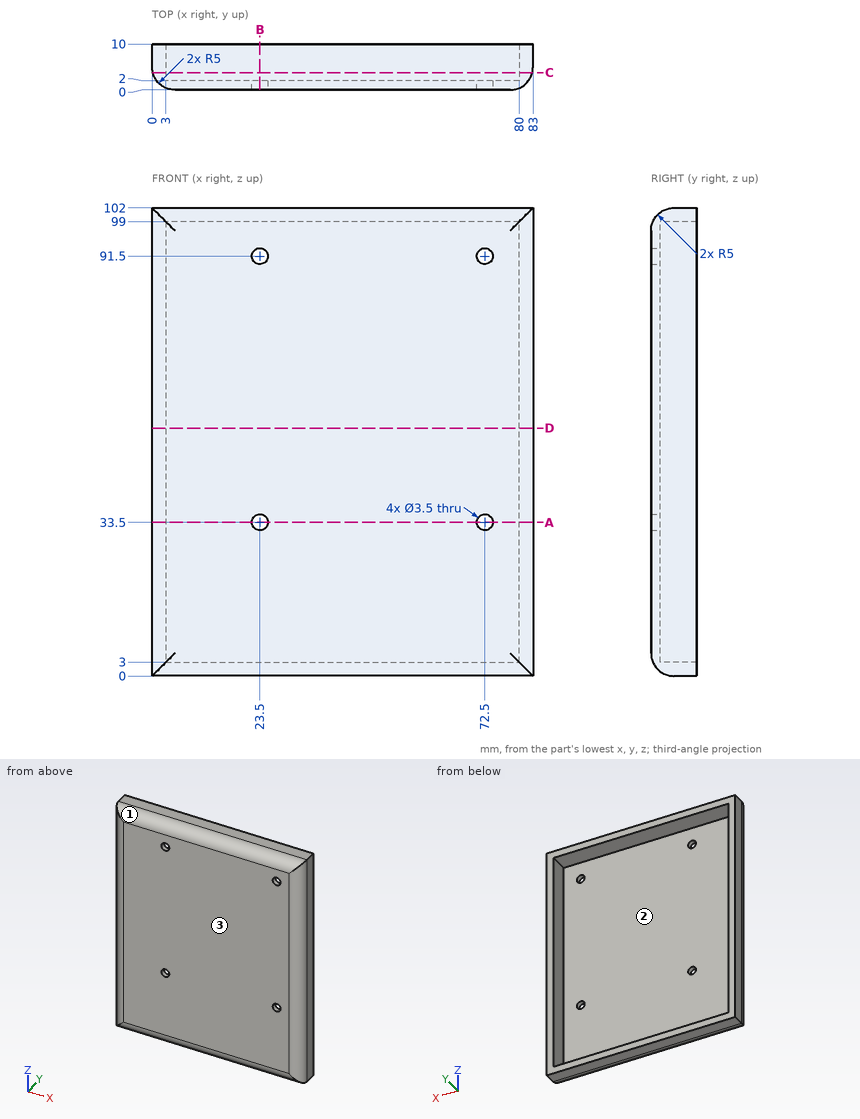
Check sheet for the drawn part. Datum: minimum x, y, z corner. Units: mm. Round coordinates to 2 decimals unless told otherwise and drop trailing zeros. Loops run counter-clockwise (first coordinate to the right, second up) from the corner with the lowest first, then second, coordinate; pieces in that order, holes last. Notation, with made-up numbers: (-2.75, 23) -> (53.25, 23) arc R36 ccw to (53.25, 62) -> close; hole circle Ø4 at (20.25, 1). An arc over 180 degrees is marked (long way). Put each result on its own line as item: value. Start each with the question number.
1. Section check B-B (x = 23.5). Enter the section's corners in (y, z), plus the area to 3 significant figures.
2. Gauge pin test, flat ends, axial feed: pin 1 (3 mm diameter, centred on x = 72.5, z = 91.5, fed in from -Y); pin 2 (5.5 mm diameter, centred on x = 23.5, z = 33.5, fed in from +Y); pin 3 (2 mm diameter, centred on y = 1, z = 86, fed in from +X); pin 4 (3 mm diameter, centred on x = 22.5, y = 3, fed in from -Z). Record the tip position at first contact, or that the pin passes through.
3. Section check D-D (z = 54). Enter the section's corners in (x, y), plus the area to 3 significant figures.
4. Section check C-C (y = 3.75). Enter the section's corners in (x, z), plus the area to 3 significant figures.
5. Draft check along Z on the marked faces 1, 2 and 3. Enter one of: +Z half, -Z half, draft (parallel to the pull), parting line (faces both ways), or undercut.
6. Scan lines: probe 1 along X at (y, z) = (7.75, 7); probe 2 along Z at (x, y) = (64, 8.75); probe 3 along Z at (x, y) = (72.5, 1.65). Record each from-to range of solid material in increasing order.
7. Section check A-A (z = 33.5). Enter the section's corners in (x, y), plus the area to 3 significant figures.
Findings:
1. outline: (0, 5) arc R5 ccw to (5, 0) -> (10, 0) -> (10, 3) -> (2, 3) -> (2, 31.75) -> (0, 31.75) -> close; (0, 35.25) -> (2, 35.25) -> (2, 89.75) -> (0, 89.75) -> close; (0, 93.25) -> (2, 93.25) -> (2, 99) -> (10, 99) -> (10, 102) -> (5, 102) arc R5 ccw to (0, 97) -> close
1. area: 227 mm^2
2. pin 1: passes through
2. pin 2: stops at y = 2
2. pin 3: stops at x = 82
2. pin 4: stops at z = 0.03
3. outline: (0, 5) arc R5 ccw to (5, 0) -> (78, 0) arc R5 ccw to (83, 5) -> (83, 10) -> (80, 10) -> (80, 2) -> (3, 2) -> (3, 10) -> (0, 10) -> close
3. area: 203 mm^2
4. outline: (0.16, 0.16) -> (82.84, 0.16) -> (82.84, 101.84) -> (0.16, 101.84) -> close; hole (3, 3) -> (80, 3) -> (80, 99) -> (3, 99) -> close
4. area: 1,020 mm^2
5. face 1: +Z half
5. face 2: undercut
5. face 3: draft
6. probe 1: x = 0 to 3, 80 to 83
6. probe 2: z = 0 to 3, 99 to 102
6. probe 3: z = 1.29 to 31.75, 35.25 to 89.75, 93.25 to 100.71
7. outline: (0, 5) arc R5 ccw to (5, 0) -> (21.75, 0) -> (21.75, 2) -> (3, 2) -> (3, 10) -> (0, 10) -> close; (25.25, 0) -> (70.75, 0) -> (70.75, 2) -> (25.25, 2) -> close; (74.25, 0) -> (78, 0) arc R5 ccw to (83, 5) -> (83, 10) -> (80, 10) -> (80, 2) -> (74.25, 2) -> close
7. area: 189 mm^2
